Can you work these out from the model? Positions are in its coordinate system, mm. A direction names the side the tool comes from. Give positions to 0.01 mm unless a question says otherwise; leave off trailing zeros. Loops run counter-clockwise (first coordinate to the right, second up) from the corner with the lowest first, then second, coordinate; pieces in that order, holes last. Notation, with made-up numbers: (-18, -5.75) - (-14, -5.75) arc R5 ccw to (-14, 0.25) - close; hole circle Ø9 at (-14.5, 61.5). An arc over 180 degrees is marked (long way). Write item = value, one per line.
from build123d import *

# Parameters (mm, degrees)
F0_W     = 90.9828
F0_H     = 4.3688
F0_W_2   = 90.17
F0_H_2   = 3.556
F1_DEPTH = 50.8
F3_DEPTH = 4.3698


with BuildPart() as f1:
    # F0 (on Top) → F1 (new body)
    with BuildSketch(Plane.XY):
        Rectangle(F0_W, F0_H)
        Rectangle(F0_W_2, F0_H_2, mode=Mode.SUBTRACT)
    extrude(amount=F1_DEPTH)

    # F2 (on face) → F3 (cut, through all)
    with BuildSketch(Plane.XZ.offset(2.1844)):
        with BuildLine():
            Line((13.7414, 50.8), (-13.7414, 50.8))
            ThreePointArc((-13.7414, 50.8), (0, 37.0586), (13.7414, 50.8))
        make_face()
    extrude(amount=-F3_DEPTH, mode=Mode.SUBTRACT)


solid = f1.part
Q1. Imagine slicing it at D-D, the plane z = 39. Write out the boundary of the cut face in (x, y) (3 decimals).
Output:
outline = (-45.491, -2.184) - (-7.042, -2.184) - (-7.042, -1.778) - (-45.085, -1.778) - (-45.085, 1.778) - (-7.042, 1.778) - (-7.042, 2.184) - (-45.491, 2.184) - close; (7.042, -2.184) - (45.491, -2.184) - (45.491, 2.184) - (7.042, 2.184) - (7.042, 1.778) - (45.085, 1.778) - (45.085, -1.778) - (7.042, -1.778) - close
Q2. Imagine slicing it at B-B, the plane x = 0. Write out the boundary of the cut face in (y, z).
Output:
outline = (-2.18, 0) - (-1.78, 0) - (-1.78, 37.06) - (-2.18, 37.06) - close; (1.78, 0) - (2.18, 0) - (2.18, 37.06) - (1.78, 37.06) - close
Q3. I need wall thicknesses on L1, parallel to Y at x = -2.5, z = 7.5; L2, parallel to X at y = 1.3, z = 40.5 (3 decimals). Which ranges of each line are inside material? Lowest first, please.
Output:
L1 = -2.18 to -1.78, 1.78 to 2.18
L2 = -45.491 to -45.085, 45.085 to 45.491
Q4. Imagine slicing it at C-C, the plane z = 30. Write out the boundary of the cut face in (x, y) (3 decimals), then the cut area to 3 significant figures.
Output:
outline = (-45.491, -2.184) - (45.491, -2.184) - (45.491, 2.184) - (-45.491, 2.184) - close; hole (-45.085, -1.778) - (45.085, -1.778) - (45.085, 1.778) - (-45.085, 1.778) - close
area = 76.8 mm2
Q5. Imagine slicing it at A-A, the plane y = 0.2. Write out the boundary of the cut face in (x, z) (3 decimals), then the cut area to 3 significant figures.
Output:
outline = (-45.491, 0) - (-45.085, 0) - (-45.085, 50.8) - (-45.491, 50.8) - close; (45.085, 0) - (45.491, 0) - (45.491, 50.8) - (45.085, 50.8) - close
area = 41.3 mm2
Q6. We'd pull the mould along Y, two halves only. Please class faces 3 (the flat face through (-1, -1.778, 25)), 4 (the flat face through (-1, 2.184, 25)), 5 (the flat face through (-45.085, 0, 25)), 6 (the cylindrical face through (-0.3, -1.98, 37.06)): released by +Y, released by -Y, zero draft, split by the parting line, or undercut.
Output:
face_3 = undercut
face_4 = released by +Y
face_5 = undercut
face_6 = zero draft
Q7. Which directions (+Z, -Z, +X, -X, +Y, -Y) give clear straight access to the entire face, cutting with the end or side of a thin tool? Please do faces 1 (the flat face through (-1, 1.778, 25)), 2 (the cylindrical face through (-0.3, 1.98, 37.06)).
Output:
face_1 = +Z, -Z
face_2 = +Z, +Y, -Y
